Build history of the part. All positions in model axes, mm. A direction names the side the tool comes from. Round coordinates to 2 decimals unless told otherwise and drop trailing zeros. Write each loop counter-clockwise with the first axis right and the second up, starting at its lowest first coordinate (ties: lowest second). Pieces come first, ordered by that corner, then holes. Notation, with made-up numbers: (17.5, -38.75) - (72.5, -38.75) arc R32 ccw to (72.5, -6.75) - close; hole circle Ø3 at (4.25, 74.5). An arc over 180 degrees is marked (long way). Answer as a JSON object with one key per item and string values. Group by question number.
Item 1: Which spindle directions (+Z, -Z, +X, -X, +Y, -Y) get a long thin tool onto all of the face, cutting with end or side? Do faces 4 (the flat face through (61, -3, -9.5)), 5 (the flat face through (9, -17.6, 22.1)), 6 (the flat face through (33, -9, -12.5)). Say none if no direction does.
Item 2: Slice it at C-C, the plane z = 19.25. List the corners of the cut face in (x, y), then the cut area to 3 significant figures.
Item 3: Flat gauge pins, fed straight in: pin 1 (1 mm diameter, centred on x = 63.5, z = 11.5, fed in from -Y); pin 2 (7 mm diameter, centred on x = 38.5, y = -15.5, fed in from +Z); pin 3 (11.5 mm diameter, centred on y = -18.5, z = 19.5, fed in from +X). Where does each tip first touch, or does it go through?
Item 4: Slice it at B-B, the plane y = -19.5. List the corners of the cut face in (x, z), then the cut area to 3 significant figures.
Item 5: Slice it at A-A, the plane z = 2.5. List the corners of the cut face in (x, y), then the cut area to 3 significant figures.
Item 6: Two-plate mould, pull along X, no slides. Class faces 1 (the cylindrical face through (56.045, -6.349, 11.537)), 2 (the cylindrical face through (43.906, -6.162, -0.263)), 3 (the flat face through (11, -1.25, -19)): +X half, -X half, draft (parallel to the pull), parting line (faces both ways), or undercut.
Item 7: Slice it at D-D, the plane x = 55. List the corners of the cut face in (y, z), then the cut area to 3 significant figures.
Item 8: Probe line 1 (Z direction, x = 2.75, y = -5.5); line 2 (X direction, y = -5.25, z = -0.5); line 3 (Y direction, x = 7, z = 20). List the from-to ranges inside material, lowest first. Write a range as from..to.
from build123d import *

# Parameters (mm, degrees)
BOSS_EXTRUDE1_DEPTH     = 12.5
SKETCH2_W               = 52
SKETCH2_H               = 25
SKETCH2_R               = 3
BOSS_EXTRUDE2_DEPTH     = 12
CUT_EXTRUDE2_DEPTH      = 75.33707016
FILLET1_R               = 2
FILLET2_R               = 3
CUT_EXTRUDE3_DEPTH      = 75.47791619
CUT_EXTRUDE3_DEPTH_BACK = 75.47791619
SKETCH7_R               = 2.75
CUT_EXTRUDE4_START      = 11
SKETCH7_3_R             = 2.75
CUT_EXTRUDE4_DEPTH      = 20
SKETCH9_W               = 8.25
SKETCH9_H               = 8.25
CUT_EXTRUDE5_DEPTH      = 3
SKETCH12_W              = 8.5
SKETCH12_H              = 8.5
CUT_EXTRUDE7_DEPTH      = 3
FILLET3_R               = 3


with BuildPart() as part:
    # Sketch1 → Boss-Extrude1 (new, symmetric)
    with BuildSketch(Plane.XY):
        Polygon((12, -25), (33, -12.5), (65, -12.5), (65, 0), (0, 0), (0, -25), align=None)
    extrude(amount=BOSS_EXTRUDE1_DEPTH, both=True)

    # Sketch2 → Boss-Extrude2 (add)
    with BuildSketch(Plane.ZY):
        with Locations((0, -12.5)):
            Rectangle(SKETCH2_W, SKETCH2_H)
        with Locations(Location((-19.25, -5.5, 0), (0, 0, 270))):
            Circle(SKETCH2_R, mode=Mode.SUBTRACT)
        with Locations(Location((-19.25, -19.5, 0), (0, 0, 270))):
            Circle(SKETCH2_R, mode=Mode.SUBTRACT)
        with Locations(Location((19.25, -19.5, 0), (0, 0, 270))):
            Circle(SKETCH2_R, mode=Mode.SUBTRACT)
        with Locations(Location((19.25, -5.5, 0), (0, 0, 270))):
            Circle(SKETCH2_R, mode=Mode.SUBTRACT)
    extrude(amount=-BOSS_EXTRUDE2_DEPTH)

    # Sketch4 → Cut-Extrude2 (cut, through all)
    with BuildSketch(Plane(origin=(0, 0, 0), x_dir=(1, 0, 0), z_dir=(0, 1, 0))):
        with BuildLine():
            Line((56.086871117, -0.4), (65, -0.4))
            Line((65, -0.4), (65, 0.4))
            Line((65, 0.4), (56.086871117, 0.4))
            ThreePointArc((56.086871117, 0.4), (43.9, 0), (56.086871117, -0.4))
        make_face()
    extrude(amount=-CUT_EXTRUDE2_DEPTH, mode=Mode.SUBTRACT)

    # Fillet1
    fillet1_edges = [part.edges().sort_by_distance(p)[0] for p in [
        (6, -25, -26),
        (6, 0, -26),
        (6, 0, 26),
        (6, -25, 26),
    ]]
    fillet(fillet1_edges, radius=FILLET1_R)

    # Fillet2
    fillet2_edges = [part.edges().sort_by_distance(p)[0] for p in [
        (65, -6.25, 12.5),
        (65, -6.25, -12.5),
    ]]
    fillet(fillet2_edges, radius=FILLET2_R)

    # Sketch7 → Cut-Extrude3 (cut, two sides: drawn at the far end of the back side and taken through both)
    with BuildSketch(Plane.XY.offset(-0.4).offset(-CUT_EXTRUDE3_DEPTH_BACK)):
        with Locations(Location((60.543435559, -6.25, 0), (0, 0, 58.017528447))):
            Circle(SKETCH7_R)
    extrude(amount=CUT_EXTRUDE3_DEPTH + CUT_EXTRUDE3_DEPTH_BACK, mode=Mode.SUBTRACT)

    # Sketch7<3> → Cut-Extrude4 (cut)
    with BuildSketch(Plane.XY.offset(-0.4).offset(CUT_EXTRUDE4_START)):
        with Locations((60.543435559, -6.25)):
            Circle(SKETCH7_3_R)
        with BuildLine():
            Line((60.543435559, -1.75), (65, -1.75))
            Line((65, -1.75), (65, -10.75))
            Line((65, -10.75), (60.543435559, -10.75))
            ThreePointArc((60.543435559, -10.75), (56.043435559, -6.25), (60.543435559, -1.75))
        make_face()
    extrude(amount=CUT_EXTRUDE4_DEPTH, mode=Mode.SUBTRACT)

    # Sketch9 → Cut-Extrude5 (cut)
    with BuildSketch(Plane(origin=(0, 0, -12.5), x_dir=(-1, 0, 0), z_dir=(0, 0, -1))):
        with Locations((-60.543435559, -6.25)):
            Rectangle(SKETCH9_W, SKETCH9_H)
    extrude(amount=-CUT_EXTRUDE5_DEPTH, mode=Mode.SUBTRACT)

    # Sketch12 → Cut-Extrude7 (cut)
    with BuildSketch(Plane(origin=(12, 0, 0), x_dir=(0, 0, -1), z_dir=(1, 0, 0))):
        with Locations((19.25, -5.5)):
            Rectangle(SKETCH12_W, SKETCH12_H)
        with Locations((-19.25, -5.5)):
            Rectangle(SKETCH12_W, SKETCH12_H)
        with Locations((19.25, -19.5)):
            Rectangle(SKETCH12_W, SKETCH12_H)
        with Locations((-19.25, -19.5)):
            Rectangle(SKETCH12_W, SKETCH12_H)
    extrude(amount=-CUT_EXTRUDE7_DEPTH, mode=Mode.SUBTRACT)

    # Fillet3
    # the kernel refuses this fillet: 3 mm, written as the material it adds along each edge
    with BuildSketch(Plane(origin=(12, -32.5, -12.5), x_dir=(1, 0, 0), z_dir=(0, 1, 0))) as fillet3_piece_1_section:
        with BuildLine():
            CenterArc((FILLET3_R, FILLET3_R), FILLET3_R, 180, 90)
            Line((0, FILLET3_R), (0, 0))
            Line((0, 0), (FILLET3_R, 0))
        make_face()
    fillet3_piece_1 = extrude(amount=32.5, mode=Mode.PRIVATE)
    fillet3_piece_1 = split(fillet3_piece_1, bisect_by=Plane(origin=(12.672630608, -24.599624638, -13.288072161), z_dir=(-0.5114838597676827, 0.8592928844097069, 0)), keep=Keep.TOP, mode=Mode.PRIVATE)
    fillet3_piece_1 = split(fillet3_piece_1, bisect_by=Plane(origin=(12.457820622, -24.238743862, -15), z_dir=(0, 0, 1)), keep=Keep.TOP, mode=Mode.PRIVATE)
    add(fillet3_piece_1)
    with BuildSketch(Plane(origin=(12, -32.5, -12.5), x_dir=(1, 0, 0), z_dir=(0, 1, 0))) as fillet3_piece_2_section:
        with BuildLine():
            CenterArc((FILLET3_R, FILLET3_R), FILLET3_R, 180, 90)
            Line((0, FILLET3_R), (0, 0))
            Line((0, 0), (FILLET3_R, 0))
        make_face()
    fillet3_piece_2 = extrude(amount=40, mode=Mode.PRIVATE)
    fillet3_piece_2 = split(fillet3_piece_2, bisect_by=Plane(origin=(12.285585988, -24.830008341, -15.125075667), z_dir=(-0.5114838597676827, 0.8592928844097069, 0)), keep=Keep.TOP, mode=Mode.PRIVATE)
    fillet3_piece_2 = split(fillet3_piece_2, bisect_by=Plane(origin=(12.012528257, -23.75, -15.125075667), z_dir=(0, -1, 0)), keep=Keep.TOP, mode=Mode.PRIVATE)
    add(fillet3_piece_2)
    with BuildSketch(Plane(origin=(12, -32.5, -12.5), x_dir=(1, 0, 0), z_dir=(0, 1, 0))) as fillet3_piece_3_section:
        with BuildLine():
            CenterArc((FILLET3_R, FILLET3_R), FILLET3_R, 180, 90)
            Line((0, FILLET3_R), (0, 0))
            Line((0, 0), (FILLET3_R, 0))
        make_face()
    fillet3_piece_3 = extrude(amount=40, mode=Mode.PRIVATE)
    fillet3_piece_3 = split(fillet3_piece_3, bisect_by=Plane(origin=(12.012572796, -15.25, -15.124824501), z_dir=(0, 1, 0)), keep=Keep.TOP, mode=Mode.PRIVATE)
    fillet3_piece_3 = split(fillet3_piece_3, bisect_by=Plane(origin=(12.012572796, -9.75, -15.124824501), z_dir=(0, -1, 0)), keep=Keep.TOP, mode=Mode.PRIVATE)
    add(fillet3_piece_3)
    with BuildSketch(Plane(origin=(12, -32.5, -12.5), x_dir=(1, 0, 0), z_dir=(0, 1, 0))) as fillet3_piece_4_section:
        with BuildLine():
            CenterArc((FILLET3_R, FILLET3_R), FILLET3_R, 180, 90)
            Line((0, FILLET3_R), (0, 0))
            Line((0, 0), (FILLET3_R, 0))
        make_face()
    fillet3_piece_4 = extrude(amount=32.5, mode=Mode.PRIVATE)
    fillet3_piece_4 = split(fillet3_piece_4, bisect_by=Plane(origin=(12.012572796, -1.25, -15.124824501), z_dir=(0, 1, 0)), keep=Keep.TOP, mode=Mode.PRIVATE)
    add(fillet3_piece_4)
    with BuildSketch(Plane(origin=(12, -32.5, 12.5), x_dir=(1, 0, 0), z_dir=(0, 1, 0))) as fillet3_piece_5_section:
        with BuildLine():
            CenterArc((FILLET3_R, -FILLET3_R), FILLET3_R, 90, 90)
            Line((0, -FILLET3_R), (0, 0))
            Line((0, 0), (FILLET3_R, 0))
        make_face()
    fillet3_piece_5 = extrude(amount=32.5, mode=Mode.PRIVATE)
    fillet3_piece_5 = split(fillet3_piece_5, bisect_by=Plane(origin=(12.672630608, -24.599624638, 13.288072161), z_dir=(-0.5114838597676827, 0.8592928844097069, 0)), keep=Keep.TOP, mode=Mode.PRIVATE)
    fillet3_piece_5 = split(fillet3_piece_5, bisect_by=Plane(origin=(12.457820622, -24.238743862, 15), z_dir=(0, 0, -1)), keep=Keep.TOP, mode=Mode.PRIVATE)
    add(fillet3_piece_5)
    with BuildSketch(Plane(origin=(12, -32.5, 12.5), x_dir=(1, 0, 0), z_dir=(0, 1, 0))) as fillet3_piece_6_section:
        with BuildLine():
            CenterArc((FILLET3_R, -FILLET3_R), FILLET3_R, 90, 90)
            Line((0, -FILLET3_R), (0, 0))
            Line((0, 0), (FILLET3_R, 0))
        make_face()
    fillet3_piece_6 = extrude(amount=40, mode=Mode.PRIVATE)
    fillet3_piece_6 = split(fillet3_piece_6, bisect_by=Plane(origin=(12.285585988, -24.830008341, 15.125075667), z_dir=(-0.5114838597676827, 0.8592928844097069, 0)), keep=Keep.TOP, mode=Mode.PRIVATE)
    fillet3_piece_6 = split(fillet3_piece_6, bisect_by=Plane(origin=(12.012528257, -23.75, 15.125075667), z_dir=(0, -1, 0)), keep=Keep.TOP, mode=Mode.PRIVATE)
    add(fillet3_piece_6)
    with BuildSketch(Plane(origin=(12, -32.5, 12.5), x_dir=(1, 0, 0), z_dir=(0, 1, 0))) as fillet3_piece_7_section:
        with BuildLine():
            CenterArc((FILLET3_R, -FILLET3_R), FILLET3_R, 90, 90)
            Line((0, -FILLET3_R), (0, 0))
            Line((0, 0), (FILLET3_R, 0))
        make_face()
    fillet3_piece_7 = extrude(amount=40, mode=Mode.PRIVATE)
    fillet3_piece_7 = split(fillet3_piece_7, bisect_by=Plane(origin=(12.012572796, -15.25, 15.124824501), z_dir=(0, 1, 0)), keep=Keep.TOP, mode=Mode.PRIVATE)
    fillet3_piece_7 = split(fillet3_piece_7, bisect_by=Plane(origin=(12.012572796, -9.75, 15.124824501), z_dir=(0, -1, 0)), keep=Keep.TOP, mode=Mode.PRIVATE)
    add(fillet3_piece_7)
    with BuildSketch(Plane(origin=(12, -32.5, 12.5), x_dir=(1, 0, 0), z_dir=(0, 1, 0))) as fillet3_piece_8_section:
        with BuildLine():
            CenterArc((FILLET3_R, -FILLET3_R), FILLET3_R, 90, 90)
            Line((0, -FILLET3_R), (0, 0))
            Line((0, 0), (FILLET3_R, 0))
        make_face()
    fillet3_piece_8 = extrude(amount=32.5, mode=Mode.PRIVATE)
    fillet3_piece_8 = split(fillet3_piece_8, bisect_by=Plane(origin=(12.012572796, -1.25, 15.124824501), z_dir=(0, 1, 0)), keep=Keep.TOP, mode=Mode.PRIVATE)
    add(fillet3_piece_8)


solid = part.part
Geometry says:
{
 "1": {"face 4": "-Z", "face 5": "+X", "face 6": "-Z, +X, +Y, -Y"},
 "2": {"outline": "(0, -25) - (12, -25) - (12, -23.75) - (9, -23.75) - (9, -22.5) - (0, -22.5) - close; (0, -16.5) - (9, -16.5) - (9, -15.25) - (12, -15.25) - (12, -9.75) - (9, -9.75) - (9, -8.5) - (0, -8.5) - close; (0, -2.5) - (9, -2.5) - (9, -1.25) - (12, -1.25) - (12, 0) - (0, 0) - close", "area": "141 mm^2"},
 "3": {"pin 1": "stops at y = -12.5", "pin 2": "stops at z = 12.5", "pin 3": "stops at x = 12.56"},
 "4": {"outline": "(0, -26) - (12, -26) - (12, -23.5) - (9, -23.5) - (9, -22.25) - (0, -22.25) - close; (0, -16.25) - (9, -16.25) - (9, -15) - (12.04, -15) arc R3 cw to (15, -12.5) - (21.24, -12.5) - (21.24, 12.5) - (15, 12.5) arc R3 cw to (12.04, 15) - (9, 15) - (9, 16.25) - (0, 16.25) - close; (0, 22.25) - (9, 22.25) - (9, 23.5) - (12, 23.5) - (12, 26) - (0, 26) - close", "area": "700 mm^2"},
 "5": {"outline": "(0, -25) - (12, -25) - (33, -12.5) - (44.44, -12.5) - (44.44, 0) - (0, 0) - close; (55.56, -12.5) - (65, -12.5) - (65, 0) - (55.56, 0) - close; hole circle Ø5.5 at (60.54, -6.25)", "area": "931 mm^2"},
 "6": {"face 1": "+X half", "face 2": "undercut", "face 3": "draft"},
 "7": {"outline": "(-12.5, -12.5) - (0, -12.5) - (0, -3.49) - (-12.5, -3.49) - close; (-12.5, 3.49) - (0, 3.49) - (0, 12.5) - (-12.5, 12.5) - close", "area": "225 mm^2"},
 "8": {"line 1": "z = -26..-22.25, -16.25..16.25, 22.25..26", "line 2": "x = 0..43.92, 56.08..57.98, 63.11..65", "line 3": "y = -25..-22.4, -16.6..-8.4, -2.6..0"}
}
